Geometry: final body of the model. Coordinates: model frame, mm. A direction names the side the tool comes from. Round coordinates to 2 decimals unless told otherwise and drop trailing zeros. Order: outer loops, then holes, each group sorted by start corner. A loop starts at its lowest first (then second) coordinate and runs counter-clockwise, first axis right, second up. Notation, with made-up numbers: (88.5, 23.25) - (109.5, 23.25) arc R30 cw to (109.5, 51.25) - close; hole circle Ø8 at (14.25, 9.25). An arc over 180 degrees is marked (long way). Put each result on its own line as item: value. Start each with the question number.
(1) Pin query (flat end, axial travel): P1, Ø3, axis at x = -11, y = -3, coming from the +Z side; P2, Ø1.3, axis at x = -9.99, z = 0, coming from the +Y side; P3, Ø1, axis at y = -1, z = -2, coming from the -X side; P4, Ø0.7, axis at y = -0.5, z = 2, coming from the +X side. Return the tip coordinate at first contact, or that it passes through.
(2) Material intervals for L1, parallel to Y at x = -13.5, z = 0; L2, parallel to X at y = -7, z = 3.75; L3, parallel to Z at x = 14.5, y = -5, sorted ascending. Write a range as [from, to].
(3) Section A-A (x = 2.5). Output: boundary loops of the cut face in (y, z).
(4) Section C-C (z = 0). Count the separate pieces of the cut face and the enclosed holes in it, and give its area (3 significant figures).
(5) Access query for faces 4 (the face through (0, -3, 10.414)), 5 (the face through (0, -1, -7.938)), 6 (the face through (14.5, -3.43, -0.65)). Directions: +Z, -Z, +X, -X, +Y, -Y. A direction counts if a zero-diameter tool reaches every point of the face in a straight line with its end or side. Return the directions, or none.
(6) Pull-direction query (Z, two-part tool) for faces 1 (the face through (7.62, -1, 0)), 2 (the face through (1.1, -3.34, 10.88)), 3 (the face through (0.1, -3.5, -10.6)); classes: released by +Z, released by -Z, zero draft, split by the parting line, or undercut.
(7) Section B-B (y = -7.75). Output: boundary loops of the cut face in (x, z), and give its area (3 significant figures).
from build123d import *
from build123d import SkipClean  # not in build123d's __all__

# Parameters (mm, degrees)
F0_R           = 1.0795
F1_DEPTH       = 2
F3_DEPTH       = 19.9898
F4_R           = 0.508
F5_R           = 0.6
F6_DEPTH       = 28.0045
F7_R           = 1.7
F7_R_2         = 0.6
F8_DEPTH       = 1.016
F9_R           = 1.7
F9_R_2         = 0.6
F10_DEPTH      = 1.016
F12_DEPTH      = 25.4
F12_DEPTH_BACK = 25.4


# Not quite as in the source:
# - after a boolean that leaves OpenCascade's solid faulty, fix() repairs it


with BuildPart() as f1:
    # F0 (on Front) → F1 (new body)
    with BuildSketch(Plane.XZ):
        with BuildLine():
            Line((8.92175, 11.43), (-8.92175, 11.43))
            ThreePointArc((-8.92175, 11.43), (-12.5138524484, 9.9421024484), (-14.00175, 6.35))
            Line((-14.00175, 6.35), (-14.00175, -6.35))
            ThreePointArc((-14.00175, -6.35), (-12.5138524484, -9.9421024484), (-8.92175, -11.43))
            Line((-8.92175, -11.43), (8.92175, -11.43))
            ThreePointArc((8.92175, -11.43), (12.5138524484, -9.9421024484), (14.00175, -6.35))
            Line((14.00175, -6.35), (14.00175, 6.35))
            ThreePointArc((14.00175, 6.35), (12.5138524484, 9.9421024484), (8.92175, 11.43))
        make_face()
        with Locations((-9.9949, 0)):
            Circle(F0_R, mode=Mode.SUBTRACT)
        with BuildLine():
            ThreePointArc((-7.62, 5.9055), (-7.0248409794, 7.3423409794), (-5.588, 7.9375))
            Line((-5.588, 7.9375), (5.588, 7.9375))
            ThreePointArc((5.588, 7.9375), (7.0248409794, 7.3423409794), (7.62, 5.9055))
            Line((7.62, 5.9055), (7.62, -5.9055))
            ThreePointArc((7.62, -5.9055), (7.0248409794, -7.3423409794), (5.588, -7.9375))
            Line((5.588, -7.9375), (-5.588, -7.9375))
            ThreePointArc((-5.588, -7.9375), (-7.0248409794, -7.3423409794), (-7.62, -5.9055))
            Line((-7.62, -5.9055), (-7.62, 5.9055))
        make_face(mode=Mode.SUBTRACT)
        with Locations((9.9949, 0)):
            Circle(F0_R, mode=Mode.SUBTRACT)
    extrude(amount=F1_DEPTH)

    # F2 (on face) → F3 (join)
    with BuildSketch(Plane.XZ.offset(2)):
        with BuildLine():
            Line((8.92175, 11.43), (-8.92175, 11.43))
            ThreePointArc((-8.92175, 11.43), (-12.5138524484, 9.9421024484), (-14.00175, 6.35))
            Line((-14.00175, 6.35), (-14.00175, -6.35))
            ThreePointArc((-14.00175, -6.35), (-12.5138524484, -9.9421024484), (-8.92175, -11.43))
            Line((-8.92175, -11.43), (8.92175, -11.43))
            ThreePointArc((8.92175, -11.43), (12.5138524484, -9.9421024484), (14.00175, -6.35))
            Line((14.00175, -6.35), (14.00175, 6.35))
            ThreePointArc((14.00175, 6.35), (12.5138524484, 9.9421024484), (8.92175, 11.43))
        make_face()
        with BuildLine():
            ThreePointArc((-12.98575, 4.064), (-11.1258780605, 8.5541280605), (-6.63575, 10.414))
            Line((-6.63575, 10.414), (6.63575, 10.414))
            ThreePointArc((6.63575, 10.414), (11.1258780605, 8.5541280605), (12.98575, 4.064))
            Line((12.98575, 4.064), (12.98575, -4.064))
            ThreePointArc((12.98575, -4.064), (11.1258780605, -8.5541280605), (6.63575, -10.414))
            Line((6.63575, -10.414), (-6.63575, -10.414))
            ThreePointArc((-6.63575, -10.414), (-11.1258780605, -8.5541280605), (-12.98575, -4.064))
            Line((-12.98575, -4.064), (-12.98575, 4.064))
        make_face(mode=Mode.SUBTRACT)
    extrude(amount=F3_DEPTH)

    # F4
    f4_edges = [f1.edges().sort_by_distance(p)[0] for p in [
        (-11.125878, -2, -8.554128),
        (-12.98575, -2, 0),
        (-11.125878, -2, 8.554128),
        (0, -2, 10.414),
        (11.125878, -2, 8.554128),
        (12.98575, -2, 0),
        (11.125878, -2, -8.554128),
        (0, -2, -10.414),
        (-11.0744, -2, 0),
        (-7.62, -2, 0),
        (-7.024841, -2, -7.342341),
        (-7.024841, -2, 7.342341),
        (0, -2, -7.9375),
        (0, -2, 7.9375),
        (7.024841, -2, -7.342341),
        (7.024841, -2, 7.342341),
        (7.62, -2, 0),
        (8.9154, -2, 0),
    ]]
    fillet(f4_edges, radius=F4_R)

    # F5 (on face) → F6 (cut, through all)
    with BuildSketch(Plane.YZ.offset(14.00175)):
        with Locations((-5, 0)):
            Circle(F5_R)
        with Locations((-11, 0)):
            Circle(F5_R)
    extrude(amount=-F6_DEPTH, mode=Mode.SUBTRACT)

    # F7 (on face) → F8 (join)
    with BuildSketch(Plane.YZ.offset(14.00175)):
        with Locations((-5, 0)):
            Circle(F7_R)
        with Locations((-5, 0)):
            Circle(F7_R_2, mode=Mode.SUBTRACT)
        with Locations((-11, 0)):
            Circle(F7_R)
        with Locations((-11, 0)):
            Circle(F7_R_2, mode=Mode.SUBTRACT)
    extrude(amount=F8_DEPTH)

    # F9 (on face) → F10 (join)
    with BuildSketch(Plane(origin=(-14.00175, 0, 0), x_dir=(0, -1, 0), z_dir=(-1, 0, 0))):
        with Locations((11, 0)):
            Circle(F9_R)
        with Locations((11, 0)):
            Circle(F9_R_2, mode=Mode.SUBTRACT)
        with Locations((5, 0)):
            Circle(F9_R)
        with Locations((5, 0)):
            Circle(F9_R_2, mode=Mode.SUBTRACT)
    with SkipClean():  # cleaning this boolean's faces spoils the solid; the shape is the same uncleaned
        extrude(amount=F10_DEPTH)

    # F11 (on Right) → F12 (cut, two sides)
    with BuildSketch(Plane.YZ) as f12_sk:
        with BuildLine():
            ThreePointArc((-8.4645346278, -2.00025), (-9.0005, 0), (-8.4645346278, 2.00025))
            Line((-8.4645346278, 2.00025), (-2.2869158186, 12.7001996474))
            Line((-2.2869158186, 12.7001996474), (-49.9461684498, 19.8914812337))
            Line((-49.9461684498, 19.8914812337), (-49.9461684498, -23.9422454613))
            Line((-49.9461684498, -23.9422454613), (4.2036823583, -23.9422454613))
            Line((4.2036823583, -23.9422454613), (-8.4645346278, -2.00025))
        make_face()
    extrude(amount=-F12_DEPTH, mode=Mode.SUBTRACT)
    extrude(f12_sk.sketch, amount=F12_DEPTH_BACK, mode=Mode.SUBTRACT)

    add(f1.part.fix(), mode=Mode.REPLACE)


solid = f1.part
Checks:
1. P1: stops at z = 11.4
1. P2: passes through
1. P3: stops at x = -14
1. P4: stops at x = 14
2. L1: y = [-9, -5.6], [-4.4, 0]
2. L2: x = [-14, -12.99], [12.99, 14]
2. L3: z = [-1.7, -0.6], [0.6, 1.7]
3. outline: (-3.61, -10.41) - (-3.02, -11.43) - (0, -11.43) - (0, -7.94) - (-1.49, -7.94) arc R0.51 ccw to (-2, -8.45) - (-2, -9.91) arc R0.51 cw to (-2.51, -10.41) - close; (-3.61, 10.41) - (-2.51, 10.41) arc R0.51 cw to (-2, 9.91) - (-2, 8.45) arc R0.51 ccw to (-1.49, 7.94) - (0, 7.94) - (0, 11.43) - (-3.02, 11.43) - close
4. separate pieces: 6
4. enclosed holes: 0
4. area: 32.9 mm²
5. face 4: -Y
5. face 5: +Y, -Y
5. face 6: +X
6. face 1: undercut
6. face 2: released by +Z
6. face 3: released by -Z
7. outline: (-14, -3.24) - (-12.99, -3.24) - (-12.99, 3.24) - (-14, 3.24) - close; (12.99, -3.24) - (14, -3.24) - (14, 3.24) - (12.99, 3.24) - close
7. area: 13.2 mm²
